Geometry check sheet. Reference: drawing and pictorial views, mm from the part's lowest x, y, z. A direction names the side the tool comes from. Give positions to 0.01 mm unless a question says otherwise; leave off trailing zeros. Order: outer loops, then holes, each group sorted by start corner. A loop starts at its lowest first (then second) coordinate and runs counter-clockwise, first axis right, second up.
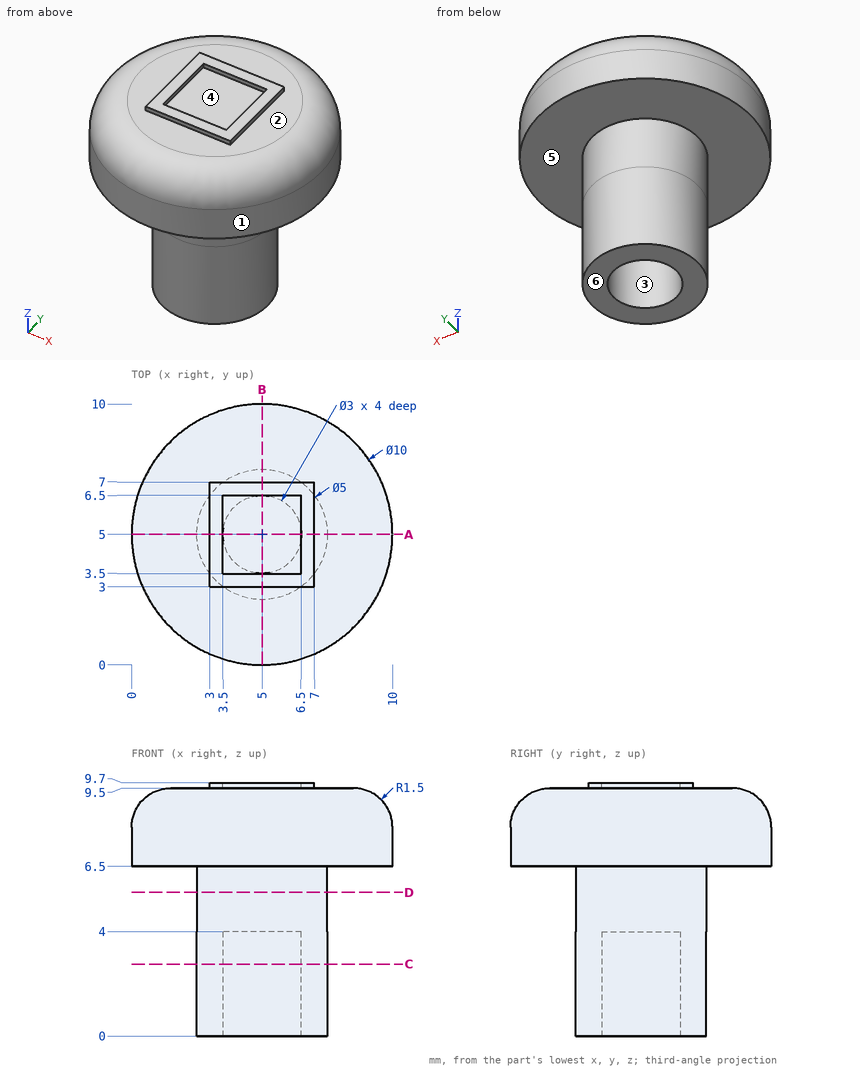
(1) Set-up check for the marked faces 4, 5 and 6: record each of +Z, -Z, +X, -X, +Y, -Y from which the full face is reachable in a straight line by a thin tool's end or side.
Response values:
face 4: +Z
face 5: -Z
face 6: -Z, +X, -X, +Y, -Y
(2) Cross-section at A-A on y = 5. Enter the section's corners in (x, z), then the cut area to 3 significant figures.
Response values:
outline: (0, 6.5) - (2.5, 6.5) - (2.5, 0) - (3.5, 0) - (3.5, 4) - (6.5, 4) - (6.5, 0) - (7.5, 0) - (7.5, 6.5) - (10, 6.5) - (10, 8) arc R1.5 ccw to (8.5, 9.5) - (7, 9.5) - (7, 9.7) - (6.5, 9.7) - (6.5, 9.5) - (3.5, 9.5) - (3.5, 9.7) - (3, 9.7) - (3, 9.5) - (1.5, 9.5) arc R1.5 ccw to (0, 8) - close
area: 49.7 mm2
(3) Material ranges on L1, parallel to Y at x = 5, z = 3; L2, parallel to Y at x = 3.75, z = 3, recorded low to high.
Response values:
L1: y = 2.5 to 3.5, 6.5 to 7.5
L2: y = 2.83 to 4.17, 5.83 to 7.17
(4) Release check for a two-part mould opening along Y. For the marked faces 1, 2 and 3 record: released by +Y, released by -Y, zero draft, split by the parting line, or undercut.
Response values:
face 1: split by the parting line
face 2: zero draft
face 3: undercut
(5) Cross-section at C-C on z = 2.75. Enter the section's corners in (x, y).
Response values:
outline: circle Ø5 at (5, 5); hole circle Ø3 at (5, 5)
(6) Cross-section at D-D on z = 5.5. Enter the section's corners in (x, y).
Response values:
outline: circle Ø5 at (5, 5)
(7) Gauge pin test, flat ends, axial feed: pin 1 Ø5 at (x, z) = (6, 2) entering from -Y; pin 2 Ø1 at (x, y) = (8, 6) entering from -Z; pin 3 Ø1 at (y, z) = (5.5, 1.5) entering from -X. Record the tip position at first contact, or that the pin passes through.
Response values:
pin 1: stops at y = 2.5
pin 2: stops at z = 6.5
pin 3: stops at x = 2.5
